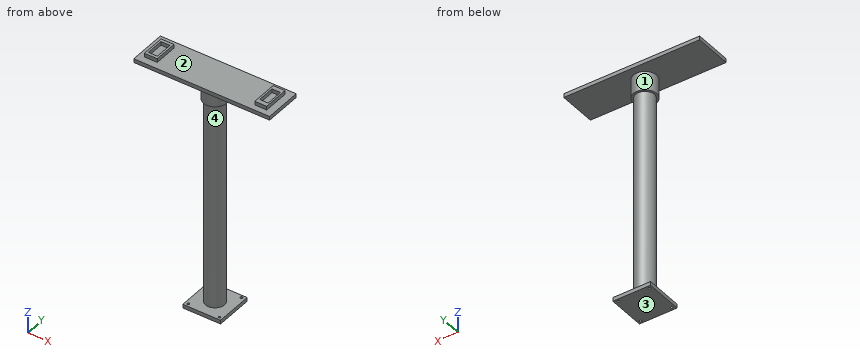
```python
from build123d import *

# Parameters (mm, degrees)
F0_W      = 254
F0_H      = 254
F0_R      = 7.765626
F0_R_2    = 62.44742
F1_DEPTH  = 25.4
F2_R      = 63.5
F3_DEPTH  = 1524
F4_R      = 63.5
F5_DEPTH  = 25.4
F4_W      = 914.4
F4_H      = 254
F6_DEPTH  = 25.4
F8_W      = 79.844535
F8_H      = 175.243094
F8_W_2    = 57.27005
F8_H_2    = 118.286156
F9_W      = 79.844535
F9_H      = 175.243094
F9_W_2    = 57.27005
F9_H_2    = 118.286156
F9_W_3    = 45.544207
F9_H_3    = 10.561109
F10_DEPTH = 25.4
F11_W     = 86.844683
F11_H     = 159.707428
F11_W_2   = 61.185301
F11_H_2   = 120.797262
F12_DEPTH = 25.4
F13_R     = 77.71217
F14_DEPTH = 127


with BuildPart() as f1:
    # F0 (on Top) → F1 (new body)
    with BuildSketch(Plane.XY):
        Rectangle(F0_W, F0_H)
        with Locations((-104.70859, -106.652051)):
            Circle(F0_R, mode=Mode.SUBTRACT)
        with Locations((106.550232, -108.094081)):
            Circle(F0_R, mode=Mode.SUBTRACT)
        with Locations((-106.150627, 106.76983)):
            Circle(F0_R, mode=Mode.SUBTRACT)
        Circle(F0_R_2, mode=Mode.SUBTRACT)
        with Locations((101.503089, 108.93289)):
            Circle(F0_R, mode=Mode.SUBTRACT)
        Circle(F0_R_2)
    extrude(amount=F1_DEPTH)

    # F2 (on face) → F3 (join)
    with BuildSketch(Plane.XY.offset(25.4)):
        Circle(F2_R)
    extrude(amount=F3_DEPTH)

    # F4 (on face) → F5 (join)
    with BuildSketch(Plane.XY.offset(1549.4)):
        Circle(F4_R)
    extrude(amount=F5_DEPTH)

    # F4 (on face) → F6 (join)
    with BuildSketch(Plane.XY.offset(1549.4)):
        Rectangle(F4_W, F4_H)
        Circle(F4_R, mode=Mode.SUBTRACT)
    extrude(amount=F6_DEPTH)

    # F8 (on face) + F9 (on face) → F10 (join)
    with BuildSketch(Plane.XY.offset(1574.8)):
        with Locations((369.877309, 0)):
            Rectangle(F8_W, F8_H)
        with Locations((370.58115, 0)):
            Rectangle(F8_W_2, F8_H_2, mode=Mode.SUBTRACT)
    with BuildSketch(Plane.XY.offset(1574.8)):
        with Locations((369.877309, 0)):
            Rectangle(F9_W, F9_H)
        with Locations((370.58115, 0)):
            Rectangle(F9_W_2, F9_H_2, mode=Mode.SUBTRACT)
        with Locations((371.858775, 73.884032)):
            Rectangle(F9_W_3, F9_H_3, mode=Mode.SUBTRACT)
    extrude(amount=F10_DEPTH)

    # F11 (on face) → F12 (join)
    with BuildSketch(Plane.XY.offset(1574.8)):
        with Locations((-375.767172, 0)):
            Rectangle(F11_W, F11_H)
        with Locations((-375.767172, 0)):
            Rectangle(F11_W_2, F11_H_2, mode=Mode.SUBTRACT)
    extrude(amount=F12_DEPTH)

    # F13 (on face) → F14 (join)
    with BuildSketch(Plane.XY.offset(1549.4)):
        Circle(F13_R)
    extrude(amount=-F14_DEPTH)


solid = f1.part
```
Geometry: final body of the model. Coordinates: model frame, mm. Face numbers are marked on the shaded views. A direction names the side the tool comes from. Round coordinates to 2 decimals unless told otherwise and drop trailing zeros. Loops run counter-clockwise (first coordinate to the right, second up) from the corner with the lowest first, then second, coordinate; pieces in that order, holes last. Notation, with made-up numbers: (84, -23.5) -> (94, -23.5) arc R25 cw to (94, -1.5) -> close; hole circle Ø10 at (41, 7.25). An arc over 180 degrees is marked (long way). Use one line per item in the form item = value. Start each with the question number.
1) First-contact query: P1, Ø12.5, axis at y = 10, z = 1584.5, coming from the -X side; P2, Ø2, axis at x = 231.5, y = -63.5, coming from the +Z side; P3, Ø20.5, axis at x = -386, z = 1587.5, coming from the -Y side. Flat tips, straight axial feed; report the tip coordinate or a pass-through.
2) Section D-D on x = -290.5. Output: boundary loops of the cut face in (y, z).
3) Draft query along Y for the marked faces 1 and 2. Return one class per face: released by +Y, released by -Y, zero draft, split by the parting line, or undercut.
4) Section C-C on z = 863.5. Output: boundary loops of the cut face in (x, y).
5) Section B-B on x = 0. Output: boundary loops of the cut face in (y, z).
6) Line query: L1, parallel to Z at x = -86, y = 98; L2, parallel to Z at x = -58, y = 40.5; L3, parallel to Z at x = -169, y = -95. Output: solid intervals per line, ascending.
7) Access query for the marked faces 3 and 4. Directions: +Z, -Z, +X, -X, +Y, -Y. A direction counts if a zero-diameter tool reaches every point of the face in a straight line with its end or side. Return the directions, or none.
Response:
q1.P1 = -419.19
q1.P2 = 1574.8
q1.P3 = -79.85
q2.outline = (-127, 1549.4) -> (127, 1549.4) -> (127, 1574.8) -> (-127, 1574.8) -> close
q3.face_1 = split by the parting line
q3.face_2 = zero draft
q4.outline = circle Ø127 at (0, 0)
q5.outline = (-127, 0) -> (127, 0) -> (127, 25.4) -> (63.5, 25.4) -> (63.5, 1422.4) -> (77.71, 1422.4) -> (77.71, 1549.4) -> (127, 1549.4) -> (127, 1574.8) -> (-127, 1574.8) -> (-127, 1549.4) -> (-77.71, 1549.4) -> (-77.71, 1422.4) -> (-63.5, 1422.4) -> (-63.5, 25.4) -> (-127, 25.4) -> close
q6.L1 = 0 to 25.4, 1549.4 to 1574.8
q6.L2 = 0 to 25.4, 1422.4 to 1574.8
q6.L3 = 1549.4 to 1574.8
q7.face_3 = -Z, +X, -X, +Y, -Y
q7.face_4 = none
